Here's how the part is built. I have some questions about the finished solid (model axes, mm). Face numbers are marked on the shaded views. A direction names the side the tool comes from. Coordinates: 2 decimals unless noted, no trailing zeros. Write each loop counter-clockwise with the first axis right and the second up, starting at its lowest first coordinate (ties: lowest second). Pieces come first, ordered by that corner, then holes.
Item 1: We'd pull the mould along Z, two halves only. Please class the marked faces 1, 2 and 3: +Z half, -Z half, draft (parallel to the pull), parting line (faces both ways), or undercut.
Item 2: If we section it at B-B (x = 55): Please give me the cut outline in (y, z).
Item 3: I'm going to push flat-ended pins straight in: pin 1 Ø0.6 at (x, y) = (77.5, 28) entering from +Z; pin 2 Ø1.6 at (x, z) = (77.5, -7.5) entering from -Y; pin 3 Ø0.6 at (x, z) = (-28.5, -56) entering from +Y. Where does each tip first touch, or does it pass through?
Item 4: If we section it at A-A (z = 2): Count the separate pieces of the cut face and the enclosed holes in it, then the cut area to 3 significant figures.
Item 5: For the marked faces 4, 5 and 6, which set-ups out of +Z, -Z, +X, -X, +Y, -Y let a thin tool reach every point of the face, with its end or its side?
Item 6: If I drill on line 1 (Z direction, x = 45.5, y = 19); line 2 (X direction, y = 32.5, z = -87.5); line 3 (Z direction, x = -49, y = 32), over which ranges is the centre line in solid material (lowest first)?
Item 7: If we section it at C-C (y = 19.5): Please give me the cut outline in (x, z), then the cut area to 3 significant figures.
Item 8: If we section it at D-D (x = 71.5): Please give me the cut outline in (y, z), then the cut area to 3 significant figures.
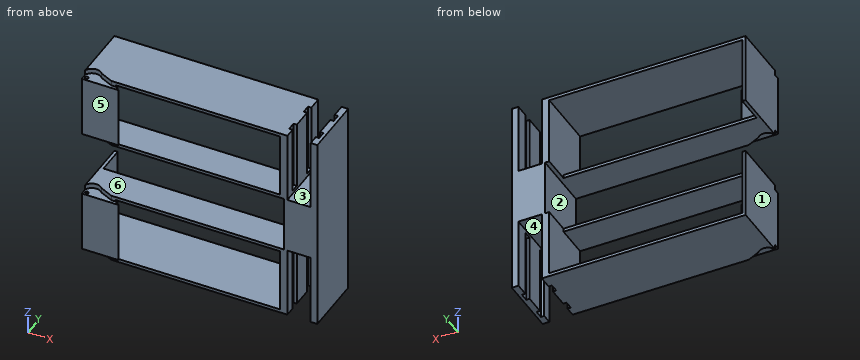
from build123d import *

# Parameters (mm, degrees)
SKETCH2_W            = 120
SKETCH2_H            = 43
BOSS_EXTRUDE1_DEPTH  = 38
SKETCH3_W            = 116
SKETCH3_H            = 39
CUT_EXTRUDE1_DEPTH   = 38
BOSS_EXTRUDE2_DEPTH  = 39
SKETCH5_W            = 43
SKETCH5_H            = 38
BOSS_EXTRUDE3_DEPTH  = 2.5
SKETCH6_W            = 2
SKETCH6_H            = 38
BOSS_EXTRUDE4_DEPTH  = 17
SKETCH7_W            = 34
SKETCH7_H            = 38
BOSS_EXTRUDE5_DEPTH  = 18
SKETCH8_W            = 4
SKETCH8_H            = 38
BOSS_EXTRUDE6_DEPTH  = 43
SKETCH9_W            = 18
SKETCH9_H            = 5
CUT_EXTRUDE2_DEPTH   = 41
SKETCH11_W           = 120
SKETCH11_H           = 2
CUT_EXTRUDE3_DEPTH   = 118.5
CUT_EXTRUDE4_DEPTH   = 3
MIRROR4_COPY_1_DEPTH = 3
CUT_EXTRUDE5_START   = -114
SKETCH13_R           = 1
CUT_EXTRUDE5_DEPTH   = 114
SKETCH14_W           = 116
SKETCH14_H           = 2
CUT_EXTRUDE6_DEPTH   = 16.6


with BuildPart() as part:
    # Sketch2 → Boss-Extrude1 (new body)
    with BuildSketch(Plane(origin=(0, 0, 0), x_dir=(1, 0, 0), z_dir=(0, 1, 0))):
        Rectangle(SKETCH2_W, SKETCH2_H)
    extrude(amount=BOSS_EXTRUDE1_DEPTH)

    # Sketch3 → Cut-Extrude1 (cut)
    with BuildSketch(Plane(origin=(0, 38, 0), x_dir=(1, 0, 0), z_dir=(0, 1, 0))):
        Rectangle(SKETCH3_W, SKETCH3_H)
    extrude(amount=-CUT_EXTRUDE1_DEPTH, mode=Mode.SUBTRACT)

    # Sketch4 → Boss-Extrude2 (add)
    with BuildSketch(Plane.XY.offset(-19.5)):
        Polygon((-58, 0), (-58, 15), (-38, 0), align=None)
    extrude(amount=BOSS_EXTRUDE2_DEPTH)

    # Sketch5 → Boss-Extrude3 (add)
    with BuildSketch(Plane(origin=(60, 0, 0), x_dir=(0, 0, -1), z_dir=(1, 0, 0))):
        with Locations((0, 19)):
            Rectangle(SKETCH5_W, SKETCH5_H)
    extrude(amount=BOSS_EXTRUDE3_DEPTH)

    # Sketch6 → Boss-Extrude4 (add)
    with BuildSketch(Plane(origin=(0, 0, -21.5), x_dir=(-1, 0, 0), z_dir=(0, 0, -1))):
        with Locations((-61.5, 19)):
            Rectangle(SKETCH6_W, SKETCH6_H)
    extrude(amount=BOSS_EXTRUDE4_DEPTH)

    # Mirror1: part across plane


with BuildPart() as part_1:
    add(part.part)
    add(part.part.mirror(Plane(origin=(0, 0, -38.5), x_dir=(1, 0, 0), z_dir=(0, 0, -1))))

    # Sketch7 → Boss-Extrude5 (add)
    with BuildSketch(Plane(origin=(62.5, 0, 0), x_dir=(0, 0, -1), z_dir=(1, 0, 0))):
        with Locations((38.5, 19)):
            Rectangle(SKETCH7_W, SKETCH7_H)
    extrude(amount=BOSS_EXTRUDE5_DEPTH)

    # Sketch8 → Boss-Extrude6 (add)
    with BuildSketch(Plane.XY.offset(-21.5)):
        with Locations((78.5, 19)):
            Rectangle(SKETCH8_W, SKETCH8_H)
    boss_extrude6 = extrude(amount=BOSS_EXTRUDE6_DEPTH)

    # Sketch9 → Cut-Extrude2 (cut)
    with BuildSketch(Plane.XY.offset(21.5)):
        with Locations((69.5, 27.5)):
            Rectangle(SKETCH9_W, SKETCH9_H)
        with Locations((69.5, 10.5)):
            Rectangle(SKETCH9_W, SKETCH9_H)
    cut_extrude2 = extrude(amount=-CUT_EXTRUDE2_DEPTH, mode=Mode.SUBTRACT)

    # Mirror2: Boss-Extrude6, Cut-Extrude2 across plane
    add(boss_extrude6.mirror(Plane(origin=(0, 0, -38.5), x_dir=(1, 0, 0), z_dir=(0, 0, -1))))
    add(cut_extrude2.mirror(Plane(origin=(0, 0, -38.5), x_dir=(1, 0, 0), z_dir=(0, 0, -1))), mode=Mode.SUBTRACT)

    # Sketch11 → Cut-Extrude3 (cut)
    with BuildSketch(Plane(origin=(80.5, 0, 0), x_dir=(0, 0, -1), z_dir=(1, 0, 0))):
        with Locations((38.5, 1)):
            Rectangle(SKETCH11_W, SKETCH11_H)
    extrude(amount=-CUT_EXTRUDE3_DEPTH, mode=Mode.SUBTRACT)

    # Sketch12 → Cut-Extrude4 (cut)
    with BuildSketch(Plane.XY.offset(21.5)):
        with BuildLine():
            Line((-38, 2), (-49.614835193, 2))
            ThreePointArc((-49.614835193, 2), (-56.018375168, 7.287996976), (-60, 0))
            Line((-60, 0), (-38, 0))
            Line((-38, 0), (-38, 2))
        make_face()
    cut_extrude4 = extrude(amount=-CUT_EXTRUDE4_DEPTH, mode=Mode.SUBTRACT)

    # Mirror3: Cut-Extrude4 across plane
    add(cut_extrude4.mirror(Plane.XY), mode=Mode.SUBTRACT)

    # Mirror4: Cut-Extrude4 across plane
    add(cut_extrude4.mirror(Plane(origin=(0, 0, -38.5), x_dir=(1, 0, 0), z_dir=(0, 0, -1))), mode=Mode.SUBTRACT)

    # Mirror4 copy 1 sketch → Mirror4 copy 1 (cut)
    with BuildSketch(Plane.XY.offset(-55.5)):
        with BuildLine():
            Line((-38, 2), (-49.614835193, 2))
            ThreePointArc((-49.614835193, 2), (-56.018375168, 7.287996976), (-60, 0))
            Line((-60, 0), (-38, 0))
            Line((-38, 0), (-38, 2))
        make_face()
    extrude(amount=-MIRROR4_COPY_1_DEPTH, mode=Mode.SUBTRACT)

    # Sketch13 → Cut-Extrude5 (cut)
    with BuildSketch(Plane.XY.offset(18.5).offset(CUT_EXTRUDE5_START)):
        with Locations((-58, 2)):
            Circle(SKETCH13_R)
    extrude(amount=CUT_EXTRUDE5_DEPTH, mode=Mode.SUBTRACT)

    # Chamfer1
    # the kernel refuses this chamfer: 10 mm, written as the material it takes off along each edge
    with BuildSketch(Plane(origin=(-49.614835193, 2, 38.180669666), x_dir=(-0.41152080336556635, 0.9114003666870882, 0), z_dir=(0, 0, -1))) as chamfer1_piece_1:
        with BuildLine():
            Line((4.024103798, 0), (-2.897424879, 6.010331734))
            Line((-2.897424879, 6.010331734), (-3.079704953, 5.928027573))
            ThreePointArc((-3.079704953, 5.928027573), (-1.554736759, 2.957293148), (-0.182280073, -0.082304161))
            Line((-0.182280073, -0.082304161), (0.082304161, -0.182280073))
            ThreePointArc((0.082304161, -0.182280073), (2.000716354, 0.27264804), (3.968173362, -0.192020276))
            Line((3.968173362, -0.192020276), (4.024103798, 0))
        make_face()
    extrude(amount=19.680669666, mode=Mode.SUBTRACT)

    # Chamfer2
    # the kernel refuses this chamfer: 10 mm, written as the material it takes off along each edge
    with BuildSketch(Plane(origin=(-49.614835193, 2, -38.180669666), x_dir=(0.9996854583228201, -0.0250795617564035, 0), z_dir=(0, 0, 1))) as chamfer2_piece_1:
        with BuildLine():
            Line((6.672267866, 0), (-1.747462586, 3.624884258))
            Line((-1.747462586, 3.624884258), (-1.896145364, 3.491117927))
            ThreePointArc((-1.896145364, 3.491117927), (-0.623209418, 1.920628258), (-0.199937092, -0.005015912))
            Line((-0.199937092, -0.005015912), (0.005015912, -0.199937092))
            ThreePointArc((0.005015912, -0.199937092), (3.339051469, -0.116294632), (6.677283779, -0.199937092))
            Line((6.677283779, -0.199937092), (6.672267866, 0))
        make_face()
    extrude(amount=19.680669666, mode=Mode.SUBTRACT)

    # Chamfer3
    # the kernel refuses this chamfer: 10 mm, written as the material it takes off along each edge
    with BuildSketch(Plane(origin=(-49.614835193, 2, -38.819330334), x_dir=(0.9996854583228201, -0.02507956175640344, 0), z_dir=(0, 0, -1))) as chamfer3_piece_1:
        with BuildLine():
            Line((6.672267866, 0), (-1.747462586, -3.624884258))
            Line((-1.747462586, -3.624884258), (-1.896145364, -3.491117927))
            ThreePointArc((-1.896145364, -3.491117927), (-0.623209418, -1.920628258), (-0.199937092, 0.005015912))
            Line((-0.199937092, 0.005015912), (0.005015912, 0.199937092))
            ThreePointArc((0.005015912, 0.199937092), (3.339051469, 0.116294632), (6.677283779, 0.199937092))
            Line((6.677283779, 0.199937092), (6.672267866, 0))
        make_face()
    extrude(amount=19.680669666, mode=Mode.SUBTRACT)

    # Chamfer4
    # the kernel refuses this chamfer: 10 mm, written as the material it takes off along each edge
    with BuildSketch(Plane(origin=(-49.614835193, 2, -115.180669666), x_dir=(0.9996854583228201, -0.0250795617564035, 0), z_dir=(0, 0, 1))) as chamfer4_piece_1:
        with BuildLine():
            Line((6.672267866, 0), (-1.747462586, 3.624884258))
            Line((-1.747462586, 3.624884258), (-1.896145364, 3.491117927))
            ThreePointArc((-1.896145364, 3.491117927), (-0.623209418, 1.920628258), (-0.199937092, -0.005015912))
            Line((-0.199937092, -0.005015912), (0.005015912, -0.199937092))
            ThreePointArc((0.005015912, -0.199937092), (3.339051469, -0.116294632), (6.677283779, -0.199937092))
            Line((6.677283779, -0.199937092), (6.672267866, 0))
        make_face()
    extrude(amount=19.680669666, mode=Mode.SUBTRACT)

    # Sketch14 → Cut-Extrude6 (cut)
    with BuildSketch(Plane(origin=(0, 38, 0), x_dir=(1, 0, 0), z_dir=(0, 1, 0))):
        with Locations((0, 20.5)):
            Rectangle(SKETCH14_W, SKETCH14_H)
    cut_extrude6 = extrude(amount=-CUT_EXTRUDE6_DEPTH, mode=Mode.SUBTRACT)

    # Mirror5: Cut-Extrude6 across plane
    add(cut_extrude6.mirror(Plane(origin=(0, 0, -38.5), x_dir=(1, 0, 0), z_dir=(0, 0, -1))), mode=Mode.SUBTRACT)


solid = part_1.part
Answer list:
1. face 1: draft
1. face 2: undercut
1. face 3: +Z half
2. outline: (2, -98.5) - (38, -98.5) - (38, -96.5) - (2, -96.5) - close; (2, -57.5) - (21.4, -57.5) - (21.4, -55.5) - (2, -55.5) - close; (2, -21.5) - (21.4, -21.5) - (21.4, -19.5) - (2, -19.5) - close; (2, 19.5) - (38, 19.5) - (38, 21.5) - (2, 21.5) - close
3. pin 1: stops at z = -19.5
3. pin 2: stops at y = 2
3. pin 3: stops at y = 21.4
4. separate pieces: 3
4. enclosed holes: 1
4. area: 489 mm2
5. face 4: -Z, +Y, -Y
5. face 5: +Z, -Z, +X, -X, -Y
5. face 6: -X, +Y, -Y
6. line 1: z = -98.5 to -96.5, -57.5 to -55.5, -21.5 to -19.5, 19.5 to 21.5
6. line 2: x = -60 to -58, 58 to 62.5, 76.5 to 80.5
6. line 3: z = -98.5 to -96.5, 19.5 to 21.5
7. outline: (-60, -98.5) - (62.5, -98.5) - (62.5, -55.5) - (76.5, -55.5) - (76.5, -98.5) - (80.5, -98.5) - (80.5, 21.5) - (76.5, 21.5) - (76.5, -21.5) - (62.5, -21.5) - (62.5, 21.5) - (-60, 21.5) - (-60, -21.5) - (60.5, -21.5) - (60.5, -55.5) - (-60, -55.5) - close; hole (-58, -96.5) - (58, -96.5) - (58, -57.5) - (-58, -57.5) - close; hole (-58, -19.5) - (58, -19.5) - (58, 19.5) - (-58, 19.5) - close
7. area: 2,510 mm2
8. outline: (2, -55.5) - (38, -55.5) - (38, -21.5) - (2, -21.5) - close
8. area: 1,220 mm2
